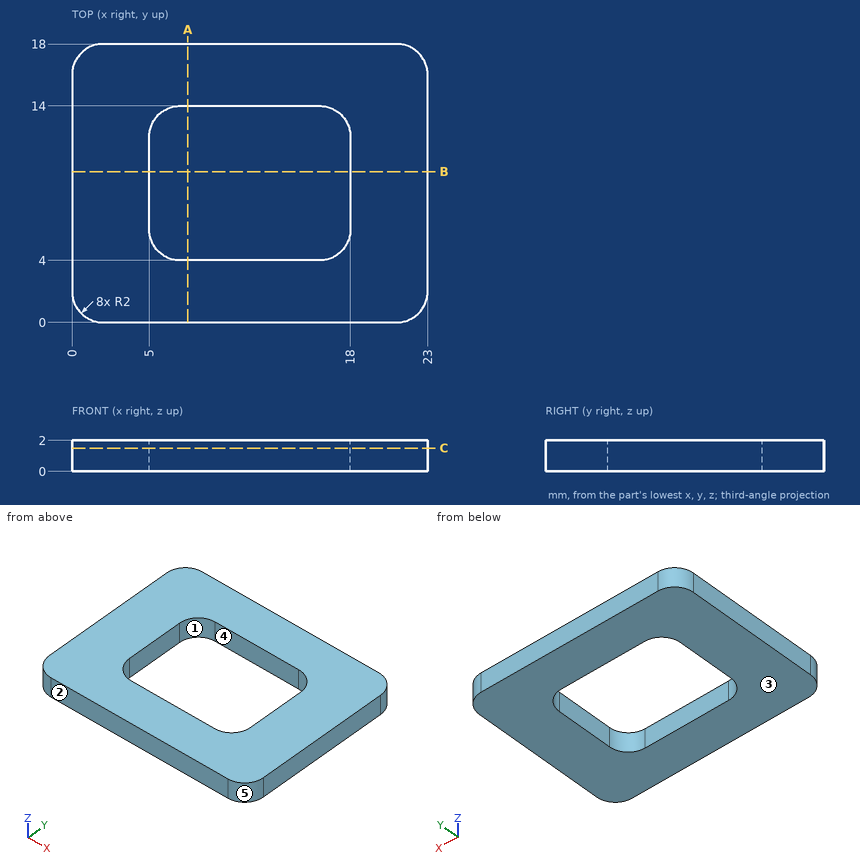
For this review, use the dimensioned drawing (mm, ordinates from the lowest corner) and the shaded views. A direction names the side the tool comes from. Round coordinates to 2 decimals unless told otherwise and drop trailing zeros. Order: outer loops, then holes, each group sorted by start corner. A loop starts at its lowest first (then second) coordinate and runs counter-clockwise, first axis right, second up. Notation, with made-up numbers: M 62.5,68.5 L 112.5,68.5 A26 ccw 112.5,104.5 Z; hole C 5.5,79.25 d4. An arc over 180 degrees is marked long. Use a Markdown table: item, result. Add a question column.
Item 1: Insertion check: pin 1 (3 mm diameter, centred on x = 17, y = 6, fed in from -Z). The pin has a flat end and moves straight along its axis. Give the tip position at first contact, or say it passes through.
Item 2: Add section A-A, the plane x = 7.5. Give the boundary of the cut face in (y, z).
Item 3: Tool access review of the marked faces 1 and 2: name each direction out of +Z, -Z, +X, -X, +Y, -Y from which nothing blocks a thin tool from reaching the whole face with its end or side.
Item 4: Add section C-C, the plane z = 1.5. Give the boundary of the cut face in (x, y), then the cut area to 3 significant figures.
Item 5: Add section B-B, the plane y = 9.75. Give the boundary of the cut face in (x, z).
Item 6: To check wall thickness, follow line 1 along Y through (x, z) = (12.75, 0.8); line 2 along X through (y, z) = (10, 1.35); line 3 along X through (y, z) = (5.25, 0.8). State the ranges of each line that lie inside material, in increasing order.
Item 7: Mouldability with a two-part tool opening along Y and no side actions: class the marked faces 3, 4 and 5 as released by +Y, released by -Y, zero draft, split by the parting line, or undercut.
Geometry results:
| question | item | result |
|---|---|---|
| 1 | pin 1 | stops at z = 0 |
| 2 | outline | M 0,0 L 4,0 L 4,2 L 0,2 Z; M 14,0 L 18,0 L 18,2 L 14,2 Z |
| 3 | face 1 | +Z, -Z |
| 3 | face 2 | +Z, -Z, +X, -X, -Y |
| 4 | outline | M 0,2 A2 ccw 2,0 L 21,0 A2 ccw 23,2 L 23,16 A2 ccw 21,18 L 2,18 A2 ccw 0,16 Z; hole M 5,6 A2 ccw 7,4 L 16,4 A2 ccw 18,6 L 18,12 A2 ccw 16,14 L 7,14 A2 ccw 5,12 Z |
| 4 | area | 284 mm² |
| 5 | outline | M 0,0 L 5,0 L 5,2 L 0,2 Z; M 18,0 L 23,0 L 23,2 L 18,2 Z |
| 6 | line 1 | y = 0 to 4, 14 to 18 |
| 6 | line 2 | x = 0 to 5, 18 to 23 |
| 6 | line 3 | x = 0 to 5.15, 17.85 to 23 |
| 7 | face 3 | zero draft |
| 7 | face 4 | undercut |
| 7 | face 5 | released by -Y |
